Can you work these out from the model? Positions are in its coordinate system, mm. A direction names the side the tool comes from. Round coordinates to 2 decimals unless told otherwise and drop trailing zeros. One line per item, written item: value. Start each with the question number.
(1) Thinking about a two-plate mould opening in X: for faces 1 (the face through (4.836, 21.241, 9.038)), 2 (the face through (-95.38, 4.44, -30.04)), 3 (the face through (-21, 10, -21)), which applies, +X half, -X half, draft (parallel to the pull), parting line (faces both ways), or undercut?
(2) I'm going to push flat-ended pins straight in: pin 1 Ø10 at (x, y) = (79, 17.5) entering from -Z; pin 2 Ø2.5 at (y, z) = (2, -26.5) entering from -X; pin 3 Ø4 at (x, y) = (0, 31.61) entering from +Z; pin 4 Ø3 at (x, y) = (-6.5, 27) entering from -Z. Where does each tip first touch, or does it pass through?
(3) On a 3-axis mill with a long thin cutter (end or side, diameter ignored), from which of +Z, -Z, +X, -X, +Y, -Y can I reach the whole of each face in a straight line? I mean faces 4 (the face through (2, 3, 5)), 5 (the face through (0, 5, -54)), 6 (the face through (-0.676, 29.463, -12.147)). Say none if no direction works.
(4) If I drill on L1, parallel to Y at x = 0, z = -12; L2, parallel to X at y = 23.5, z = 0; L3, parallel to Y at x = -92, z = -29, over which ranges is the centre line in solid material (lowest first)? Write a range as from..to.
Autodesk Inventor part; units mm, degrees
ref_plane "YZ Plane" through (0, 0, 0) normal (1, 0, 0) x (0, 1, 0)
ref_plane "XZ Plane" through (0, 0, 0) normal (0, 1, 0) x (-1, 0, 0)
ref_plane "XY Plane" through (0, 0, 0) normal (0, 0, 1) x (1, 0, 0)
sketch "Boceto2" plane through (0, 0, 0) normal (0, 1, 0) x (-1, 0, 0)
  circle A0 centre (0, 0) radius 100
  dimension "d11" = 200
extrude "Extrusión2" add sketch "Boceto2" along normal blind 10
sketch "Boceto3" plane through (0, 10, 0) normal (0, 1, 0) x (1, 0, 0)
  circle A0 centre (0, 0) radius 100
hole "Agujero1" at (0, 10, 0) direction (0, -1, 0) diameter 20.5 depth 7
sketch "Boceto4" plane through (0, 10, 0) normal (0, 1, 0) x (1, 0, 0)
  circle A0 centre (0, 0) radius 10.25
  circle A1 centre (0, 0) radius 100
  circle A2 centre (0, 0) radius 15.25
  dimension "d21" = 5
extrude "Extrusión3" add sketch "Boceto4" along normal blind 30 contours A2
sketch "Boceto5" plane through (0, 0, 0) normal (0, 0, 1) x (1, 0, 0)
  line L0 (15.25, 40) -> (-15.25, 40)
  line L1 (0, 40) -> (0, 20)
  line L2 (0, 40) -> (0, 31.6087)
  line L3 (0, 31.6087) -> (0, 23.2173)
  circle A0 centre (0, 23.2173) radius 2.25
  circle A1 centre (0, 31.6087) radius 2.25
  point P0 (0, 0)
  point P1 (-15.25, 20)
  point P2 (15.25, 20)
  dimension "d25" = 8.3913
  dimension "d26" = 8.3913
  dimension "d27" = 4.5
  dimension "d28" = 4.5
fillet "Empalme2" radius 1 1 edges at (100, 10, 0)
chamfer "Chaflán1" distance 30 angle 3 1 edges at (-15.25, 40, 0) measured on face at (15.2005, 30, 1.2271)
hole "Agujero3" at (0, 31.6087, 0) at (0, 23.2173, 0) direction (0, 0, -1) diameter 4.5 end through all
fillet "Empalme3" radius 10 2 edges at (-15.25, 10.0005, 0) (-15.25, 10, 0)
sketch "Boceto6" plane through (0, 0, 0) normal (0, -1, 0) x (1, 0, 0)
  circle A0 centre (0, 0) radius 100
  circle A1 centre (0, 0) radius 5
  line L0 (5, 0) -> (5, -105)
  line L1 (-5, 0) -> (-5, -105)
  point P0 (-5, -99.8749)
  point P1 (5, -99.8749)
  dimension "d48" = 10
  dimension "d49" = 105
  dimension "d50" = 10
extrude "Extrusión4" cut sketch "Boceto6" against normal blind 5 contours L1 A1 L0 A0 | A1 picked at (0.2009, -68.3119)
sketch "Boceto7" plane through (-5, 0, 0) normal (1, 0, 0) x (0, 0, -1)
  point P0 (0, 0)
fillet "Empalme4" radius 2 2 edges at (-5, 5, -54.4113) (5, 5, -54.4113)
properties part number "Pie2"
Established:
1. face 1: undercut
1. face 2: parting line
1. face 3: draft
2. pin 1: through
2. pin 2: x = -96.76
2. pin 3: z = 14.22
2. pin 4: z = -13.47
3. face 4: +Y
3. face 5: -Z, -Y
3. face 6: -Z
4. L1: 5..20.97, 25.47..29.36, 33.86..40
4. L2: -14.54..-10.25, 10.25..14.54
4. L3: 0..10
